```python
from build123d import *

# Parameters (mm, degrees)
SKETCH1_R                                           = 35
SKETCH1_R_2                                         = 10
BOSS_EXTRUDE1_DEPTH                                 = 30
SKETCH4_R                                           = 12.5
CUT_EXTRUDE2_DEPTH                                  = 15
CBORE_FOR_M6_HEX_SOCKET_HEAD_CAP_SCREW1_D           = 6.4
CBORE_FOR_M6_HEX_SOCKET_HEAD_CAP_SCREW1_CBORE_D     = 11
CBORE_FOR_M6_HEX_SOCKET_HEAD_CAP_SCREW1_CBORE_DEPTH = 8.4
F_8_0MM_DOWEL_HOLE1_D                               = 8
SKETCH14_OUTSIDE_W                                  = 92.688
SKETCH14_OUTSIDE_H                                  = 92.688
SKETCH14_OUTSIDE_W_2                                = 70
SKETCH14_OUTSIDE_H_2                                = 25.4
CUT_EXTRUDE3_DEPTH                                  = 2
SKETCH18_R                                          = 2.1
CUT_EXTRUDE5_DEPTH                                  = 3
CUT_EXTRUDE6_DEPTH                                  = 58.879184825
CUT_EXTRUDE6_DEPTH_BACK                             = 58.879184825
BOSS_EXTRUDE2_DEPTH                                 = 2
DRAFT1_ANGLE                                        = 3


with BuildPart() as part:
    # Sketch1 → Boss-Extrude1 (new body)
    with BuildSketch(Plane(origin=(0, 0, 0), x_dir=(1, 0, 0), z_dir=(0, 1, 0))):
        with Locations(Location((0, 0, 0), (0, 0, 270))):
            Circle(SKETCH1_R)
        with Locations(Location((0, 0, 0), (0, 0, 270))):
            Circle(SKETCH1_R_2, mode=Mode.SUBTRACT)
    extrude(amount=-BOSS_EXTRUDE1_DEPTH)

    # Sketch4 → Cut-Extrude2 (cut)
    with BuildSketch(Plane(origin=(0, 0, 0), x_dir=(1, 0, 0), z_dir=(0, 1, 0))):
        with Locations(Location((0, 0, 0), (0, 0, 270))):
            Circle(SKETCH4_R)
    extrude(amount=-CUT_EXTRUDE2_DEPTH, mode=Mode.SUBTRACT)

    # CBORE for M6 Hex Socket Head Cap Screw1 (through all)
    with Locations(Plane(origin=(0, -30, 0), x_dir=(-1, 0, 0), z_dir=(0, -1, 0))):
        with Locations((0, 25), (21.650635095, -12.5), (-21.650635095, -12.5)):
            CounterBoreHole(CBORE_FOR_M6_HEX_SOCKET_HEAD_CAP_SCREW1_D / 2, CBORE_FOR_M6_HEX_SOCKET_HEAD_CAP_SCREW1_CBORE_D / 2, CBORE_FOR_M6_HEX_SOCKET_HEAD_CAP_SCREW1_CBORE_DEPTH)

    # Ø8.0mm Dowel Hole1 (through all)
    with Locations(Plane(origin=(0, -30, 0), x_dir=(-1, 0, 0), z_dir=(0, -1, 0))):
        with Locations((13.75, -23.815698604), (-13.75, 23.815698604)):
            Hole(F_8_0MM_DOWEL_HOLE1_D / 2)

    # Sketch14 outside → Cut-Extrude3 (cut)
    with BuildSketch(Plane.XZ.offset(30)):
        Rectangle(SKETCH14_OUTSIDE_W, SKETCH14_OUTSIDE_H)
        Rectangle(SKETCH14_OUTSIDE_W_2, SKETCH14_OUTSIDE_H_2, mode=Mode.SUBTRACT)
    extrude(amount=-CUT_EXTRUDE3_DEPTH, mode=Mode.SUBTRACT)

    # Sketch18 → Cut-Extrude5 (cut)
    with BuildSketch(Plane.XZ.offset(30)):
        with Locations(Location((-13.665, 0, 0), (0, 0, 270))):
            Circle(SKETCH18_R)
    extrude(amount=-CUT_EXTRUDE5_DEPTH, mode=Mode.SUBTRACT)

    # Sketch19 → Cut-Extrude6 (cut, two sides: drawn at the far end of the back side and taken through both)
    with BuildSketch(Plane(origin=(0, 0, 0), x_dir=(0, 0, -1), z_dir=(1, 0, 0)).offset(-CUT_EXTRUDE6_DEPTH_BACK)):
        Polygon((-12.7, -28), (-12.164101615, -30), (-12.7, -30), align=None)
        Polygon((12.7, -28), (12.164101615, -30), (12.7, -30), align=None)
    extrude(amount=CUT_EXTRUDE6_DEPTH + CUT_EXTRUDE6_DEPTH_BACK, mode=Mode.SUBTRACT)

    # Sketch20 → Boss-Extrude2 (add)
    with BuildSketch(Plane.XZ.offset(30)):
        with BuildLine():
            Line((-12.581122044, 12.164101615), (12.581122044, 12.164101615))
            ThreePointArc((12.581122044, 12.164101615), (0, 17.5), (-12.581122044, 12.164101615))
        make_face()
        with BuildLine():
            Line((-12.581122044, -12.164101615), (12.581122044, -12.164101615))
            ThreePointArc((12.581122044, -12.164101615), (0, -17.5), (-12.581122044, -12.164101615))
        make_face()
    extrude(amount=-BOSS_EXTRUDE2_DEPTH)

    # Draft1
    draft1_faces = [part.faces().sort_by_distance(p)[0] for p in [
        (0, -29, -17.5),
    ]]
    draft(draft1_faces, Plane(origin=(0, -28, 0), x_dir=(0, 0, -1), z_dir=(0, -1, 0)), DRAFT1_ANGLE)


solid = part.part
```
Part model, mm, in its own coordinate system. A direction names the side the tool comes from. Round coordinates to 2 decimals unless told otherwise and drop trailing zeros. Loops run counter-clockwise (first coordinate to the right, second up) from the corner with the lowest first, then second, coordinate; pieces in that order, holes last.
Item 1: Cut at B-B, the plane z = 0. Give the cut face in (x, y) (3 decimals).
Item 2: Cut at D-D, the plane z = -25. Give the cut face in (x, y), then the cut area to 3 significant figures.
Item 3: Mould opens along X. For faces 5 (the face through (0, 0, 15)), 6 (the face through (1.539, -14.79, -34.966)), 7 (the face through (-20.174, -10.649, 15.339)) say: +X half, -X half, draft (parallel to the pull), parting line (faces both ways), or undercut.
Item 4: Cut at C-C, the plane y = -2.5. Give the cut face in (x, z).
Item 5: Drill centre lines: line 1 (X direction, y = -4, z = -23.5); line 2 (Z direction, x = 1, y = -19); line 3 (X direction, y = -25, z = 0). Where is each one in solid material? Low to high.
Item 6: 3-axis set-ups, long thin cutter, end or side, ignore diameter. For faces 1 (the face through (-2.4, -21.6, -22.6)), 2 (the face through (22.284, -28.986, -12.436)), 3 (the face through (10.2, -15, -0.1)), 4 (the face through (0.2, -29, 17.5)): which of +Z, -Z, +X, -X, +Y, -Y reach the whole face in a straight line?
Item 7: Cut at A-A, the plane x = 0. Give the cut face in (y, z).
Item 8: Drop flat-ended pins along their axis: P1, Ø2, axis at x = -10.5, y = -7, coming from the -Z side; P2, Ø2, axis at y = -16, z = -8.5, coming from the +X side; P3, Ø9, axis at x = 0, z = -25, coming from the -Y side; P4, Ø12, axis at x = -20, z = 10.5, coming from the -Y side. Give the stop position or say it passes through.
A:
1. outline: (-35, -30) - (-15.765, -30) - (-15.765, -27) - (-11.565, -27) - (-11.565, -30) - (-10, -30) - (-10, -15) - (-12.5, -15) - (-12.5, 0) - (-35, 0) - close; (10, -30) - (35, -30) - (35, 0) - (12.5, 0) - (12.5, -15) - (10, -15) - close
2. outline: (-24.49, -28) - (-5.5, -28) - (-5.5, -21.6) - (-3.2, -21.6) - (-3.2, 0) - (-24.49, 0) - close; (3.2, -21.6) - (5.5, -21.6) - (5.5, -28) - (9.93, -28) - (9.93, 0) - (3.2, 0) - close; (17.57, -28) - (24.49, -28) - (24.49, 0) - (17.57, 0) - close
2. area: 949 mm2
3. face 5: draft
3. face 6: parting line
3. face 7: undercut
4. outline: circle Ø70 at (0, 0); hole circle Ø6.4 at (-21.65, 12.5); hole circle Ø8 at (-13.75, 23.82); hole circle Ø25 at (0, 0); hole circle Ø6.4 at (0, -25); hole circle Ø8 at (13.75, -23.82); hole circle Ø6.4 at (21.65, 12.5)
5. line 1: x = -25.94 to -2.83, 2.83 to 9.76, 17.74 to 25.94
5. line 2: z = -34.99 to -28.04, -21.96 to -9.95, 9.95 to 34.99
5. line 3: x = -35 to -10, 10 to 35
6. face 1: -Y
6. face 2: -Z, +X, -Y
6. face 3: +Y
6. face 4: +Z, -Y
7. outline: (-30, -17.4) - (-28, -17.5) - (-28, -19.5) - (-21.6, -19.5) - (-21.6, -21.8) - (0, -21.8) - (0, -12.5) - (-15, -12.5) - (-15, -10) - (-30, -10) - close; (-30, 10) - (-15, 10) - (-15, 12.5) - (0, 12.5) - (0, 35) - (-28, 35) - (-28, 17.5) - (-30, 17.5) - close; (-28, -35) - (0, -35) - (0, -28.2) - (-21.6, -28.2) - (-21.6, -30.5) - (-28, -30.5) - close
8. P1: stops at z = -33.69
8. P2: stops at x = 34.19
8. P3: stops at y = -21.6
8. P4: stops at y = -30
